from build123d import *

# Parameters (mm, degrees)
SKETCH_W  = 25
SKETCH_H  = 24
SKETCH_R  = 1.35
PAD_DEPTH = 3
FILLET_R  = 1


with BuildPart() as part:
    # Sketch → Pad (new body)
    with BuildSketch(Plane.XY):
        with Locations((12.5, 12)):
            Rectangle(SKETCH_W, SKETCH_H)
        with Locations((4.1, 17)):
            Circle(SKETCH_R, mode=Mode.SUBTRACT)
        with Locations((20.1, 15)):
            Circle(SKETCH_R, mode=Mode.SUBTRACT)
        with Locations((4.1, 7)):
            Circle(SKETCH_R, mode=Mode.SUBTRACT)
        with Locations((20.1, 7)):
            Circle(SKETCH_R, mode=Mode.SUBTRACT)
    extrude(amount=PAD_DEPTH)

    # Fillet
    fillet_edges = [part.edges().sort_by_distance(p)[0] for p in [
        (0, 0, 1.5),
        (25, 0, 1.5),
        (25, 24, 1.5),
        (0, 24, 1.5),
    ]]
    fillet(fillet_edges, radius=FILLET_R)


solid = part.part
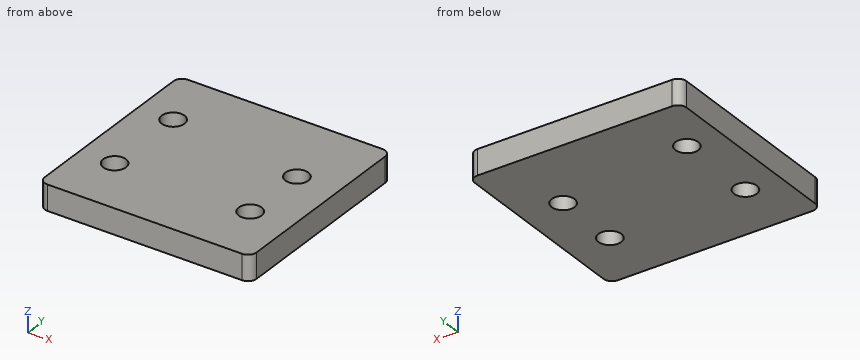
Work out the finished part from the listing and answer in its coordinate system (mm). Round coordinates to 2 decimals unless told otherwise and drop trailing zeros. Write each loop counter-clockwise with the first axis right and the second up, starting at its lowest first coordinate (ties: lowest second). Pieces come first, ordered by that corner, then holes. Notation, with made-up numbers: (-23, 19.25) -> (23, 19.25) arc R27 cw to (23, 38.25) -> close; hole circle Ø4 at (23.5, 23.5). An arc over 180 degrees is marked (long way). Answer as CSV lines item,"result". Start each with the question number.
(1) The part is cut by section D-D, the plane y = 17. Give the vertices of the cut face in (x, z), then the cut area to 3 significant figures.
(2) Find the intervals of material crossed by probe 1 along Y at (x, z) = (4.1, 2.3); probe 2 along Y at (x, z) = (20.1, 1.8); probe 3 along X at (y, z) = (7.5, 2), in increasing order.
(3) The part is cut by section B-B, the plane y = 7. Give the vertices of the cut face in (x, z).
(4) The part is cut by section A-A, the plane x = 4.1. Give the vertices of the cut face in (y, z), then the cut area to 3 significant figures.
(5) The part is cut by section C-C, the plane z = 2.3. Give the vertices of the cut face in (x, y).
Output values:
1,outline,"(0, 0) -> (2.75, 0) -> (2.75, 3) -> (0, 3) -> close; (5.45, 0) -> (25, 0) -> (25, 3) -> (5.45, 3) -> close"
1,area,"66.9 mm²"
2,probe 1,"y = 0 to 5.65, 8.35 to 15.65, 18.35 to 24"
2,probe 2,"y = 0 to 5.65, 8.35 to 13.65, 16.35 to 24"
2,probe 3,"x = 0 to 2.85, 5.35 to 18.85, 21.35 to 25"
3,outline,"(0, 0) -> (2.75, 0) -> (2.75, 3) -> (0, 3) -> close; (5.45, 0) -> (18.75, 0) -> (18.75, 3) -> (5.45, 3) -> close; (21.45, 0) -> (25, 0) -> (25, 3) -> (21.45, 3) -> close"
4,outline,"(0, 0) -> (5.65, 0) -> (5.65, 3) -> (0, 3) -> close; (8.35, 0) -> (15.65, 0) -> (15.65, 3) -> (8.35, 3) -> close; (18.35, 0) -> (24, 0) -> (24, 3) -> (18.35, 3) -> close"
4,area,"55.8 mm²"
5,outline,"(0, 1) arc R1 ccw to (1, 0) -> (24, 0) arc R1 ccw to (25, 1) -> (25, 23) arc R1 ccw to (24, 24) -> (1, 24) arc R1 ccw to (0, 23) -> close; hole circle Ø2.7 at (4.1, 7); hole circle Ø2.7 at (4.1, 17); hole circle Ø2.7 at (20.1, 7); hole circle Ø2.7 at (20.1, 15)"
